Here's how the part is built. I have some questions about the finished solid (model axes, mm). Face numbers are marked on the shaded views. A direction names the side the tool comes from. Give positions to 0.01 mm unless a question says otherwise; leave off trailing zeros. Order: outer loops, then holes, each group sorted by start corner. A loop starts at its lowest first (then second) coordinate and runs counter-clockwise, first axis right, second up.
from build123d import *

# Parameters (mm, degrees)
ESQUISSE1_R                  = 32.625
EXTRUSION1_DEPTH             = 1
ENL_V_MAT_EXTRU_1_DEPTH      = 2
R_P_TITION_CIRCULAIRE1_COUNT = 16
ESQUISSE3_R                  = 21
EXTRUSION2_DEPTH             = 2.125
ESQUISSE4_R                  = 16
ENL_V_MAT_EXTRU_2_DEPTH      = 3.125
ENL_V_MAT_EXTRU_2_DEPTH_BACK = 3.125
CHANFREIN1_SIZE              = 0.5


with BuildPart() as part:
    # Esquisse1 → Extrusion1 (new body, symmetric)
    with BuildSketch(Plane.XY):
        Circle(ESQUISSE1_R)
    extrude(amount=EXTRUSION1_DEPTH, both=True)

    # Esquisse2 → Enlèv. mat.-Extru.1 (cut, symmetric)
    with BuildSketch(Plane.XY):
        with BuildLine():
            Line((-5.281931711, 32.194593062), (-3.276608177, 29.330694255))
            ThreePointArc((-3.276608177, 29.330694255), (0.958663447, 27.741578262), (3.967875501, 31.119071146))
            Line((3.967875501, 31.119071146), (4.126482213, 32.362984559))
            ThreePointArc((4.126482213, 32.362984559), (-0.583827722, 32.619775753), (-5.281931711, 32.194593062))
        make_face()
    enl_v_mat_extru_1 = extrude(amount=ENL_V_MAT_EXTRU_1_DEPTH, both=True, mode=Mode.SUBTRACT)

    # Répétition circulaire1: Enlèv. mat.-Extru.1 ×16 about axis
    r_p_tition_circulaire1_axis = Axis((0, 0, 0), (0, 0, 1))
    for i in range(1, R_P_TITION_CIRCULAIRE1_COUNT):
        add(enl_v_mat_extru_1.rotate(r_p_tition_circulaire1_axis, i * 360 / R_P_TITION_CIRCULAIRE1_COUNT), mode=Mode.SUBTRACT)

    # Esquisse3 → Extrusion2 (add, symmetric)
    with BuildSketch(Plane.XY):
        Circle(ESQUISSE3_R)
    extrude(amount=EXTRUSION2_DEPTH, both=True)

    # Esquisse4 → Enlèv. mat.-Extru.2 (cut, two sides)
    with BuildSketch(Plane.XY) as enl_v_mat_extru_2_sk:
        Circle(ESQUISSE4_R)
    extrude(amount=ENL_V_MAT_EXTRU_2_DEPTH, mode=Mode.SUBTRACT)
    extrude(enl_v_mat_extru_2_sk.sketch, amount=-ENL_V_MAT_EXTRU_2_DEPTH_BACK, mode=Mode.SUBTRACT)

    # Chanfrein1
    chanfrein1_edges = [part.edges().sort_by_distance(p)[0] for p in [
        (-21, 0, -2.125),
        (-21, 0, 2.125),
        (-16, 0, -2.125),
        (-16, 0, 2.125),
    ]]
    chamfer(chanfrein1_edges, length=CHANFREIN1_SIZE)


solid = part.part
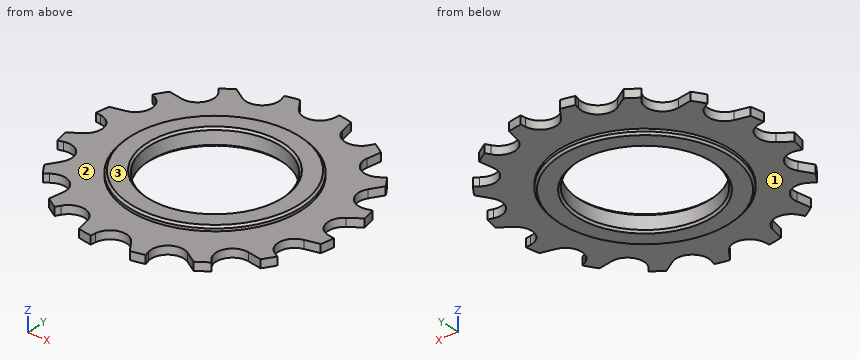
Q1. I need wall thicknesses on L1, parallel to Y at x = 0, z = 0.4 (3 decimals); L2, parallel to Y at x = 28, z = 0.3. Which ranges of each line are inside material? Lowest first, please.
Filled sheet:
L1: y = -27.625 to -16, 16 to 27.625
L2: y = -16.74 to -16.01, -8.29 to -1.69, 1.69 to 8.29
Q2. If we section it at A-A on y = 0: List the corners of the cut face in (x, z) for me (3 decimals).
Filled sheet:
outline: (-27.625, -1) - (-21, -1) - (-21, -1.625) - (-20.5, -2.125) - (-16.5, -2.125) - (-16, -1.625) - (-16, 1.625) - (-16.5, 2.125) - (-20.5, 2.125) - (-21, 1.625) - (-21, 1) - (-27.625, 1) - close; (16, -1.625) - (16.5, -2.125) - (20.5, -2.125) - (21, -1.625) - (21, -1) - (27.625, -1) - (27.625, 1) - (21, 1) - (21, 1.625) - (20.5, 2.125) - (16.5, 2.125) - (16, 1.625) - close
Q3. I'm going to push flat-ended pins straight in: P1, Ø1, axis at x = 3, z = -1, coming from the -Y side; P2, Ø3, axis at x = -24, y = -2, coming from the -Z side. Where does each tip first touch, or does it pass through?
Filled sheet:
P1: stops at y = -29.65
P2: stops at z = -1
Q4. For the marked faces 1, 2 and 3, which set-ups out of +Z, -Z, +X, -X, +Y, -Y let a thin tool reach every point of the face, with its end or its side?
Filled sheet:
face 1: -Z
face 2: +Z
face 3: +Z, +X, -X, +Y, -Y
